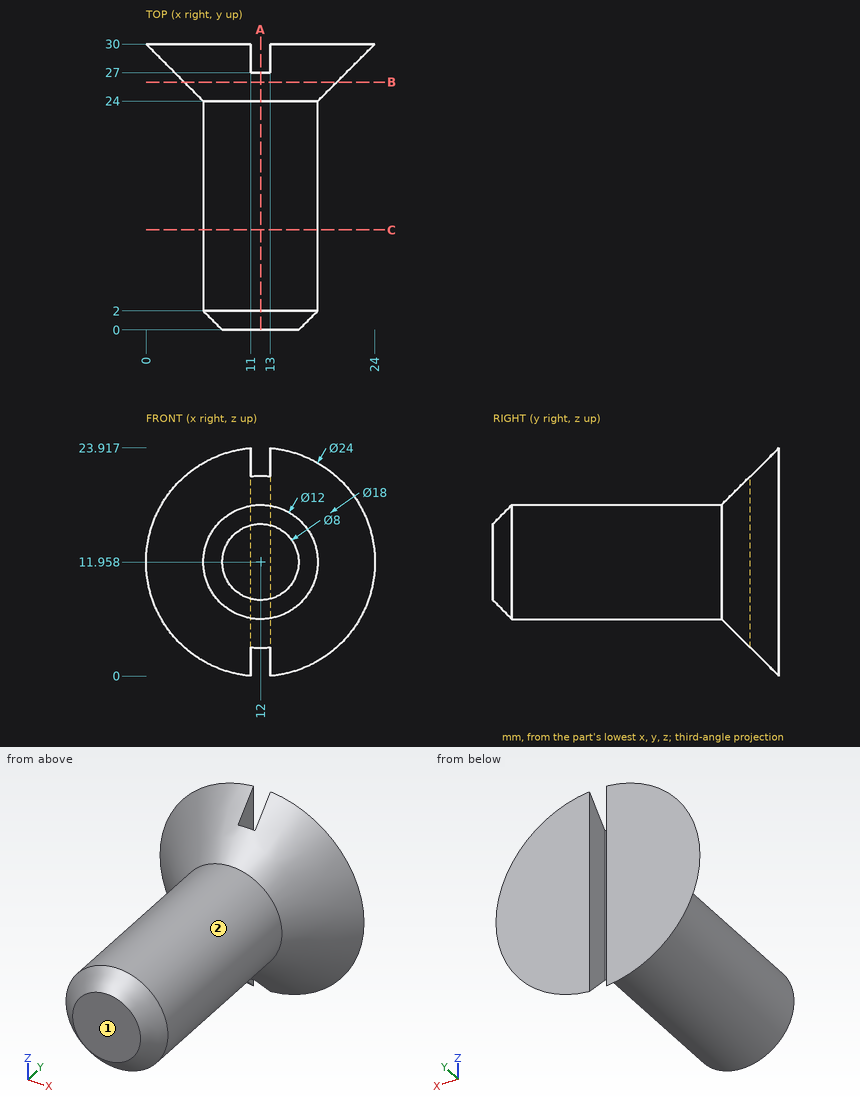
Can you work these out from the drawing? Everything is in mm from the part's minimum corner. A direction names the side the tool comes from. Coordinates: 2 decimals unless noted, no trailing zeros. Loops run counter-clockwise (first coordinate to the right, second up) from the corner with the lowest first, then second, coordinate; pieces in that order, holes last. Notation, with made-up numbers: M 37,58.5 L 90,58.5 A18 ccw 90,84.5 Z; hole C -8.75,26.5 d9. An arc over 180 degrees is marked long. One line per item, written item: value.
1. Imagine slicing it at A-A (x = 12). List the corners of the cut face in (y, z) for me, and give its area (3 significant figures).
Geometry says:
outline: M 0,7.96 L 2,5.96 L 24,5.96 L 27,2.96 L 27,20.96 L 24,17.96 L 2,17.96 L 0,15.96 Z
area: 329 mm2
2. Please list where these lines run through material, in increasing order: probe 1 along Y at (x, z) = (12.25, 9.25); probe 2 along X at (y, z) = (29.5, 7) (1 decimal); probe 3 along Z at (x, y) = (15.5, 23) (1 decimal).
Geometry says:
probe 1: y = 0 to 27
probe 2: x = 1.6 to 11, 13 to 22.4
probe 3: z = 7.1 to 16.8
3. Imagine slicing it at C-C (y = 10.5). List the corners of the cut face in (x, z) for me, and give its area (3 significant figures).
Geometry says:
outline: C 12,11.96 d12
area: 113 mm2
4. On a 3-axis mill with a long thin cutter (end or side, diameter ignored), from which of +Z, -Z, +X, -X, +Y, -Y can I reach the whole of each face in a straight line? I mean the marked faces 1 and 2. Say none if no direction works.
Geometry says:
face 1: +Z, -Z, +X, -X, -Y
face 2: -Y
5. Will these pins go through, and if not, where does the flat tip stop? pin 1 Ø2 at (y, z) = (7.5, 6.5) entering from +X (1 decimal); pin 2 Ø1.5 at (y, z) = (18.5, 3.5) entering from +X; pin 3 Ø1 at (x, y) = (12.5, 17) entering from +Z; pin 4 Ø3.5 at (y, z) = (28.5, 13) entering from -X.
Geometry says:
pin 1: stops at x = 16
pin 2: passes through
pin 3: stops at z = 17.96
pin 4: stops at x = 0
6. Imagine slicing it at B-B (y = 26). List the corners of the cut face in (x, z) for me, and give its area (3 significant figures).
Geometry says:
outline: C 12,11.96 d16
area: 201 mm2
